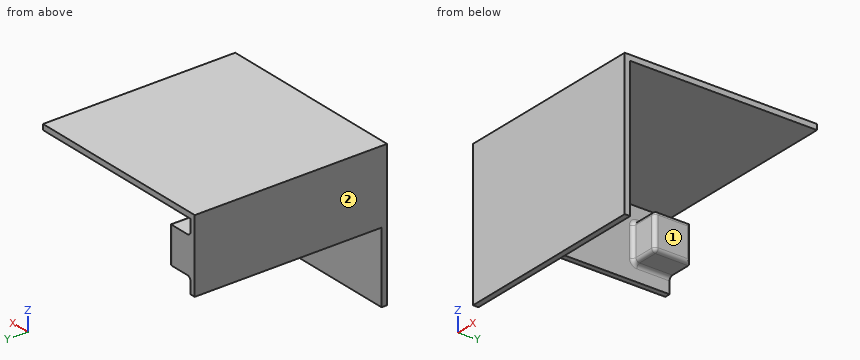
from build123d import *

# Parameters (mm, degrees)
SKETCH1_W                = 100
SKETCH1_H                = 73
BOSS_EXTRUDE1_DEPTH      = 3
BOSS_EXTRUDE2_DEPTH      = 102.5
BOSS_EXTRUDE2_DEPTH_BACK = 3
SKETCH2_W                = 106
SKETCH2_H                = 79
SKETCH2_W_2              = 100
SKETCH2_H_2              = 73
SKETCH3_W                = 106
SKETCH3_H                = 102.5
CUT_EXTRUDE1_DEPTH       = 39
CUT_EXTRUDE2_REACH       = 156.682
SKETCH4_W                = 37
SKETCH4_H                = 102.5
SKETCH5_W                = 20
SKETCH5_H                = 20
BOSS_EXTRUDE3_DEPTH      = 15
FILLET1_R                = 2


with BuildPart() as part:
    # Sketch1 → Boss-Extrude1 (new body)
    with BuildSketch(Plane(origin=(0, 0, 0), x_dir=(1, 0, 0), z_dir=(0, 1, 0))):
        Rectangle(SKETCH1_W, SKETCH1_H)
    extrude(amount=BOSS_EXTRUDE1_DEPTH)

    # Sketch2 → Boss-Extrude2 (add, two sides: drawn at the far end of the back side and taken through both)
    with BuildSketch(Plane(origin=(0, 3, 0), x_dir=(1, 0, 0), z_dir=(0, 1, 0)).offset(-BOSS_EXTRUDE2_DEPTH_BACK)):
        Rectangle(SKETCH2_W, SKETCH2_H)
        Rectangle(SKETCH2_W_2, SKETCH2_H_2, mode=Mode.SUBTRACT)
    extrude(amount=BOSS_EXTRUDE2_DEPTH + BOSS_EXTRUDE2_DEPTH_BACK)

    # Sketch3 → Cut-Extrude1 (cut)
    with BuildSketch(Plane(origin=(0, 0, -39.5), x_dir=(-1, 0, 0), z_dir=(0, 0, -1))):
        with Locations((0, 54.25)):
            Rectangle(SKETCH3_W, SKETCH3_H)
    extrude(amount=-CUT_EXTRUDE1_DEPTH, mode=Mode.SUBTRACT)

    # Sketch4 → Cut-Extrude2 (cut, up to next)
    with BuildSketch(Plane(origin=(53, 0, 0), x_dir=(0, 0, -1), z_dir=(1, 0, 0)), mode=Mode.PRIVATE) as cut_extrude2_sk1:
        with Locations((-18, 54.25)):
            Rectangle(SKETCH4_W, SKETCH4_H)
    cut_extrude2_tool1 = extrude(cut_extrude2_sk1.sketch, amount=-CUT_EXTRUDE2_REACH, mode=Mode.PRIVATE) & part.part
    add(cut_extrude2_tool1.solids().sort_by_distance((53, 54.25, 18))[0], mode=Mode.SUBTRACT)

    # Sketch5 → Boss-Extrude3 (add)
    with BuildSketch(Plane(origin=(-50, 0, 0), x_dir=(0, 0, -1), z_dir=(1, 0, 0))):
        with Locations((-18, 95.5)):
            Rectangle(SKETCH5_W, SKETCH5_H)
    extrude(amount=BOSS_EXTRUDE3_DEPTH)

    # Fillet1
    fillet1_edges = [part.edges().sort_by_distance(p)[0] for p in [
        (-50, 95.5, 8),
        (-42.5, 85.5, 8),
        (-50, 95.5, 28),
        (-50, 85.5, 18),
        (-42.5, 85.5, 28),
        (-35, 95.5, 8),
        (-35, 105.5, 18),
        (-35, 95.5, 28),
        (-35, 85.5, 18),
    ]]
    fillet(fillet1_edges, radius=FILLET1_R)


solid = part.part
Check sheet for the modelled part. Datum: model origin and axes. Units: mm. Face numbers are marked on the shaded views. A direction names the side the tool comes from. Round coordinates to 2 decimals unless told otherwise and drop trailing zeros. Order: outer loops, then holes, each group sorted by start corner. A loop starts at its lowest first (then second) coordinate and runs counter-clockwise, first axis right, second up.
(1) Scan lines: probe 1 along Y at (x, z) = (-46, 11.5); probe 2 along Z at (x, y) = (-44, 65.5); probe 3 along Y at (x, z) = (31, 13.5). Record each from-to range of solid material in increasing order.
(2) Cross-section at B-B, the plane y = 89. Enter the section's corners in (x, z).
(3) Cross-section at D-D, the plane y = 70. Enter the section's corners in (x, z), and give its area (3 significant figures).
(4) Cross-section at C-C, the plane x = 12. Enter the section's corners in (y, z), and give its area (4 significant figures).
(5) Go/stop test with flat-tipped pins: P1, Ø3, axis at x = 11.5, z = 20, coming from the +Y side; P2, Ø1, axis at x = -0.5, y = 20, coming from the -Z side; P3, Ø12, axis at x = -42.5, y = 100.5, coming from the -Z side. Record where each tip stops, or that it passes through.
(6) Access from +Z, -Z, +X, -X, +Y, -Y to the whole of each face (thin tool, end or side, straight path). Record for the marked faces 1 and 2.
(7) Cross-section at A-A, the plane z = 22. Enter the section's corners in (x, y).
Check sheet entries:
1. probe 1: y = 0 to 3, 85.5 to 105.5
1. probe 2: z = 36.5 to 39.5
1. probe 3: y = 0 to 3
2. outline: (-53, -0.5) - (-50, -0.5) - (-50, 6) arc R2 cw to (-48, 8) - (-37, 8) arc R2 ccw to (-35, 10) - (-35, 26) arc R2 ccw to (-37, 28) - (-48, 28) arc R2 cw to (-50, 30) - (-50, 36.5) - (53, 36.5) - (53, 39.5) - (-53, 39.5) - close
3. outline: (-53, -0.5) - (-50, -0.5) - (-50, 36.5) - (53, 36.5) - (53, 39.5) - (-53, 39.5) - close
3. area: 429 mm2
4. outline: (0, -39.5) - (3, -39.5) - (3, 36.5) - (105.5, 36.5) - (105.5, 39.5) - (0, 39.5) - close
4. area: 544.5 mm2
5. P1: stops at y = 3
5. P2: stops at z = 36.5
5. P3: stops at z = 7.94
6. face 1: -Z, +X, +Y
6. face 2: +Z, -Z, -X, +Y, -Y
7. outline: (-53, 0) - (53, 0) - (53, 3) - (-50, 3) - (-50, 83.5) arc R2 cw to (-48, 85.5) - (-37, 85.5) arc R2 ccw to (-35, 87.5) - (-35, 103.5) arc R2 ccw to (-37, 105.5) - (-53, 105.5) - close
